Can you work these out from the model? Positions are in its coordinate system, mm. Give positions to 0.01 mm unless a question says otherwise; leave off trailing zeros. Order: outer loops, then holes, each group sorted by start corner. A loop starts at its lowest first (then second) coordinate and runs counter-clockwise, first axis right, second up. Notation, with made-up numbers: M 59.5,82 L 66.5,82 A31 cw 66.5,119 Z; hole C 27,-0.5 d11. An arc over 180 degrees is marked long. Write each question's results on one line, items separated by ' | '.
Autodesk Fusion 360 part; units mm, degrees
sketch "Skizze1" plane through (0, 0, 0) normal (0, 1, 0) x (1, 0, 0)
  ellipse E0 centre (19.0444, -49.1025) end of major axis (19.0444, -50.6334) minor radius 1.5307
  line L0 (55.2123, -43.6898) -> (55.2123, -85.3711)
  line L1 (55.2123, -85.3711) -> (13.531, -85.3711)
  line L2 (13.531, -85.3711) -> (13.531, -43.6898)
  line L3 (13.531, -43.6898) -> (55.2123, -43.6898)
  line L4 (26.9008, -1.7518) -> (30.0736, -4.9062)
  line L5 (30.0736, -4.9062) -> (30.0582, -31.0654)
  line L6 (30.0582, -31.0654) -> (30.1165, -31.0654)
  line L7 (30.1165, -31.0654) -> (30.1165, -42.123)
  line L8 (30.1165, -42.123) -> (63.94, -42.1236)
  line L9 (63.94, -42.1236) -> (67.115, -45.2984)
  line L10 (67.115, -45.2984) -> (67.115, -83.7656)
  line L11 (67.115, -83.7656) -> (63.94, -86.9404)
  line L12 (63.94, -86.9404) -> (4.096, -86.9404)
  line L13 (4.096, -86.9404) -> (0.9212, -83.7656)
  line L14 (0.9212, -83.7656) -> (0.9212, -4.9266)
  line L15 (0.9212, -4.9266) -> (4.0757, -1.7518)
  line L16 (4.0757, -1.7518) -> (26.9008, -1.7518)
  line L17 (-656.5386, -196.3597) -> (-656.5386, -172.9852) construction
  line L18 (-656.5386, -172.9852) -> (-663.2077, -172.9852) construction
  line L19 (-663.2077, -172.9852) -> (-663.2077, -196.3597) construction
  line L20 (-663.2077, -196.3597) -> (-656.5386, -196.3597) construction
  line L21 (-786.7672, -196.3598) -> (-786.7672, -172.9853) construction
  line L22 (-786.7672, -172.9853) -> (-793.4364, -172.9853) construction
  line L23 (-793.4364, -172.9853) -> (-793.4364, -196.3598) construction
  line L24 (-793.4364, -196.3598) -> (-786.7672, -196.3598) construction
  circle A0 centre (50.0444, -49.1025) radius 1.5 construction
  circle A1 centre (50.0444, -80.1025) radius 1.5 construction
  line L25 (50.0444, -80.1025) -> (19.0444, -80.1025) construction
  circle A2 centre (19.0444, -80.1025) radius 1.5 construction
  line L26 (19.0444, -80.1025) -> (19.0444, -49.1025) construction
  circle A3 centre (34.4717, -64.6752) radius 12.5 construction
  circle A4 centre (61.4704, -49.0847) radius 1.5 construction
  circle A5 centre (61.4704, -80.2249) radius 1.5 construction
  circle A6 centre (5.4074, -7.8253) radius 1.5 construction
  circle A7 centre (25.4061, -7.8253) radius 1.5 construction
  circle A8 centre (25.4061, -22.5328) radius 1.5 construction
  circle A9 centre (5.4074, -22.5328) radius 1.5 construction
  point P0 (51.8121, -49.1024)
  point P1 (51.6713, -79.7501)
  point P2 (19.0448, -81.2802)
  point P3 (19.0444, -50.6334)
  point P4 (34.1696, -76.3823)
  point P5 (27.8065, -7.8253)
  point P6 (27.8065, -22.5328)
  point P7 (7.8078, -7.8253)
  point P8 (7.8078, -22.5328)
  point P9 (10.9547, -80.1317)
  point P10 (10.9547, -48.9915)
  point P11 (63.8708, -80.2249)
  point P12 (63.8708, -49.0847)
  dimension "d1" = 31
  dimension "d2" = 3
  dimension "d4" = 3
  dimension "d5" = 31
  dimension "d6" = 3
  dimension "d7" = 25
  dimension "d8" = 3
  dimension "d9" = 3
  dimension "d10" = 3
  dimension "d11" = 3
  dimension "d12" = 3
  dimension "d13" = 3
extrude "Extrusion1" add sketch "Skizze1" along normal blind 4 contours L0 L1 L2 L3 | L4 L5 L6 L7 L8 L9 L10 L11 L12 L13 L14 L15 L16
sketch "Skizze2" plane through (0, 4, 0) normal (0, 1, 0) x (-1, 0, 0)
  ellipse E0 centre (-19.0444, 49.1025) end of major axis (-19.0444, 50.6334) minor radius 1.5307
  line L0 (-4.0757, 1.7518) -> (-0.9212, 4.9266)
  line L1 (-0.9212, 4.9266) -> (-0.9212, 83.7656)
  line L2 (-0.9212, 83.7656) -> (-4.096, 86.9404)
  line L3 (-4.096, 86.9404) -> (-63.94, 86.9404)
  line L4 (-63.94, 86.9404) -> (-67.115, 83.7656)
  line L5 (-67.115, 83.7656) -> (-67.115, 45.2984)
  line L6 (-67.115, 45.2984) -> (-63.94, 42.1236)
  line L7 (-63.94, 42.1236) -> (-30.1165, 42.123)
  line L8 (-30.1165, 42.123) -> (-30.1165, 31.0654)
  line L9 (-30.1165, 31.0654) -> (-30.0582, 31.0654)
  line L10 (-30.0582, 31.0654) -> (-30.0736, 4.9062)
  line L11 (-30.0736, 4.9062) -> (-26.9008, 1.7518)
  line L12 (-26.9008, 1.7518) -> (-4.0757, 1.7518)
  circle A0 centre (-50.0444, 49.1025) radius 1.5
  circle A1 centre (-50.0444, 80.1025) radius 1.5
  circle A2 centre (-19.0444, 80.1025) radius 1.5
  circle A3 centre (-34.5444, 64.6025) radius 12.5
  circle A4 centre (-5, 8) radius 1.5
  circle A5 centre (-25, 8) radius 1.5
  circle A6 centre (-5, 23) radius 1.5
  circle A7 centre (-25, 23) radius 1.5
  circle A8 centre (-63, 49) radius 1.5
  circle A9 centre (-63, 78) radius 1.5
  dimension "d16" = 31
  dimension "d17" = 3
  dimension "d18" = 31
  dimension "d19" = 3
  dimension "d20" = 31
  dimension "d21" = 3
  dimension "d22" = 25
  dimension "d23" = 3
  dimension "d24" = 3
  dimension "d25" = 3
  dimension "d26" = 15
  dimension "d27" = 3
  dimension "d28" = 3
  dimension "d29" = 3
extrude "Extrusion2" cut sketch "Skizze2" against normal blind 28 contours A0 | A1 | A2 | A3 | A4 | A5 | A6 | A7 | A8 | A9
sketch "Skizze3" plane through (0, 0, 0) normal (0, 1, 0) x (1, 0, 0)
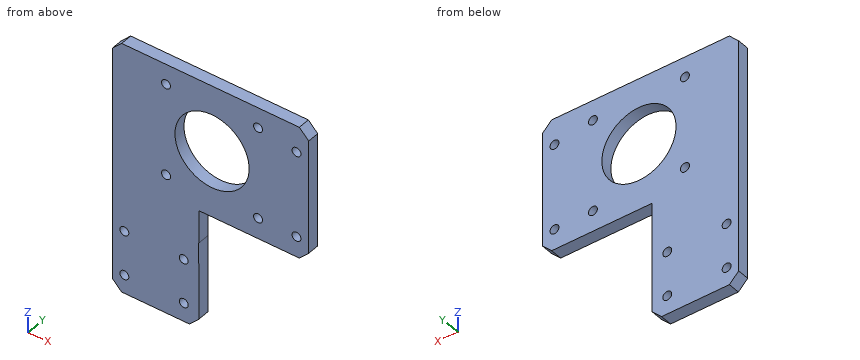
(1) I need wall thicknesses on L1, parallel to Z at x = 5, y = 2.6; L2, parallel to Z at x = 63, y = 2.7; L3, parallel to Z at x = 57.5, y = 2.5. Which ranges of each line are inside material? Lowest first, please. Write a range as from..to.
Data:
L1: z = 1.75..6.5, 9.5..21.5, 24.5..86.94 | L2: z = 42.12..47.5, 50.5..76.5, 79.5..86.94 | L3: z = 42.12..86.94
(2) Imagine slicing it at C-C, the plane x = 25. Write out the boundary of the cut face in (y, z), plus the area to 3 significant figures.
Data:
outline: M 0,1.75 L 4,1.75 L 4,6.5 L 0,6.5 Z; M 0,9.5 L 4,9.5 L 4,21.5 L 0,21.5 Z; M 0,24.5 L 4,24.5 L 4,56.53 L 0,56.53 Z; M 0,72.67 L 4,72.67 L 4,86.94 L 0,86.94 Z | area: 252 mm2
(3) Imagine slicing it at B-B, the plane z = 57.5. Write out the boundary of the cut face in (x, y) (3 decimals), plus the area to 3 significant figures.
Data:
outline: M 0.921,0 L 24.258,0 L 24.258,4 L 0.921,4 Z; M 44.831,0 L 67.115,0 L 67.115,4 L 44.831,4 Z | area: 182 mm2
(4) Imagine slicing it at D-D, the plane z = 8. Write out the boundary of the cut face in (x, y), plus the area to 3 significant figures.
Data:
outline: M 0.92,0 L 3.5,0 L 3.5,4 L 0.92,4 Z; M 6.5,0 L 23.5,0 L 23.5,4 L 6.5,4 Z; M 26.5,0 L 30.07,0 L 30.07,4 L 26.5,4 Z | area: 92.6 mm2
(5) Will these pins go through, and if not, where does the flat tip stop? P1, Ø2, axis at y = 2.5, z = 38.5, coming from the +X side; P2, Ø1.5, axis at x = 55, y = 3, coming from the -Z side; P3, Ø2.5, axis at x = 19.04, z = 80.1, coming from the +Y side.
Data:
P1: stops at x = 30.12 | P2: stops at z = 42.12 | P3: passes through
(6) Imagine slicing it at A-A, the plane x = 5. Write out the boundary of the cut face in (y, z).
Data:
outline: M 0,1.75 L 4,1.75 L 4,6.5 L 0,6.5 Z; M 0,9.5 L 4,9.5 L 4,21.5 L 0,21.5 Z; M 0,24.5 L 4,24.5 L 4,86.94 L 0,86.94 Z
